CAD build for the part. Positions are in the model's coordinates, mm. Face numbers are marked on the shaded views. A direction names the side the tool comes from. Give positions to 0.01 mm unless a question says otherwise; leave off trailing zeros. Order: outer loops, then holes, each group sorted by start corner. A loop starts at its lowest first (then second) coordinate and runs counter-clockwise, first axis right, second up. Notation, with made-up numbers: (21, -1.75) -> (46, -1.75) arc R19 cw to (46, 21.25) -> close; hole circle Ø6 at (-7.75, 21). An arc over 180 degrees is marked (long way). Use one line per item in the form item = value. Start each with the question number.
1) Drop flat-ended pins along their axis: P1, Ø3, axis at x = 2, y = 8, coming from the -Z side (3 decimals); P2, Ø5, axis at x = 3.5, z = 61, coming from the +Y side; P3, Ø10, axis at y = -8, z = 22.5, coming from the +X side. Give the stop position or say it passes through.
2) Cut at D-D, the plane x = -9.25. Give the cut face in (y, z) (3 decimals).
3) Tool access for the marked faces 1, 2 and 3: list every direction of +Z, -Z, +X, -X, +Y, -Y with a clear straight run to the whole face (end or side of a thin tool).
4) Cut at C-C, the plane z = 24.5. Give the cut face in (x, y) (1 decimal), and give its area (3 significant figures).
5) Cut at B-B, the plane y = 0. Give the cut face in (x, z) (1 decimal).
6) Probe line 1 (Z direction, x = -2, y = 4.5) (3 decimals); line 2 (Z direction, x = -6.5, y = 0.5) (3 decimals); line 3 (Y direction, x = 0.5, z = 11.5). List the from-to ranges inside material, lowest first.
7) Cut at A-A, the plane x = 0. Give the cut face in (y, z) (1 decimal), and give its area (3 significant figures).
from build123d import *

# Parameters (mm, degrees)
F0_R     = 11.1125
F1_DEPTH = 76.2
F2_R     = 15.748
F3_DEPTH = 9.525
F4_R     = 6
F5_DEPTH = 25.4
F6_R     = 6
F6_R_2   = 4.8895
F7_DEPTH = 2.794
F8_W     = 13.440132
F8_H     = 49.0506
F9_DEPTH = 85.726


with BuildPart() as f1:
    # F0 (on Top) → F1 (new body)
    with BuildSketch(Plane.XY):
        Circle(F0_R)
    extrude(amount=F1_DEPTH)

    # F2 (on face) → F3 (join)
    with BuildSketch(Plane(origin=(0, 0, 0), x_dir=(1, 0, 0), z_dir=(0, 0, -1))):
        Circle(F2_R)
    extrude(amount=F3_DEPTH)

    # F4 (on face) → F5 (join)
    with BuildSketch(Plane(origin=(0, 0, -9.525), x_dir=(1, 0, 0), z_dir=(0, 0, -1))):
        Circle(F4_R)
    extrude(amount=F5_DEPTH)

    # F6 (on face) → F7 (cut)
    with BuildSketch(Plane(origin=(0, 0, -9.525), x_dir=(1, 0, 0), z_dir=(0, 0, -1))):
        Circle(F6_R)
        Circle(F6_R_2, mode=Mode.SUBTRACT)
    extrude(amount=F7_DEPTH, mode=Mode.SUBTRACT)

    # F8 (on face) → F9 (cut, through all)
    with BuildSketch(Plane(origin=(0, 0, -9.525), x_dir=(1, 0, 0), z_dir=(0, 0, -1))):
        with Locations((-19.420066, 0)):
            Rectangle(F8_W, F8_H)
        with Locations((19.420066, 0)):
            Rectangle(F8_W, F8_H)
    extrude(amount=-F9_DEPTH, mode=Mode.SUBTRACT)


solid = f1.part
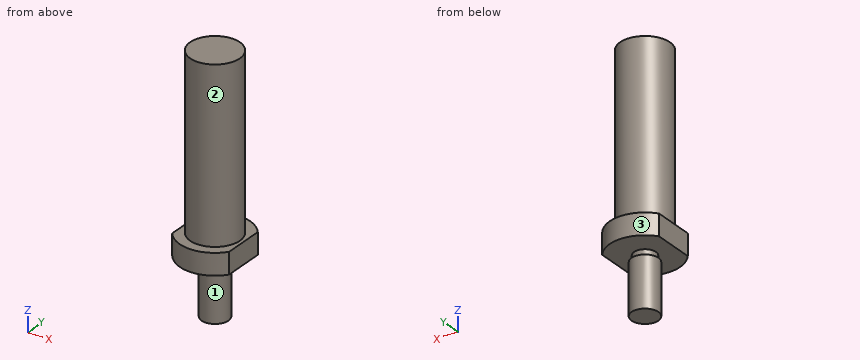
Result:
q1.P1 = -9.525
q1.P2 = 11.07
q1.P3 = 10.7
q2.outline = (-12.745, -9.525) -> (12.745, -9.525) -> (12.745, 0) -> (6.158, 0) -> (6.158, 76.2) -> (-6.158, 76.2) -> (-6.158, 0) -> (-12.745, 0) -> close
q3.face_1 = -Z
q3.face_2 = +Z
q3.face_3 = +Z, -Z, +Y
q4.outline = circle Ø22.2 at (0, 0)
q4.area = 388 mm²
q5.outline = (-12.7, -9.5) -> (-4.9, -9.5) -> (-4.9, -12.3) -> (-6, -12.3) -> (-6, -34.9) -> (6, -34.9) -> (6, -12.3) -> (4.9, -12.3) -> (4.9, -9.5) -> (12.7, -9.5) -> (12.7, 0) -> (11.1, 0) -> (11.1, 76.2) -> (-11.1, 76.2) -> (-11.1, 0) -> (-12.7, 0) -> close
q6.line_1 = -34.925 to -12.319, -9.525 to 76.2
q6.line_2 = -9.525 to 76.2
q6.line_3 = -11.1 to 11.1
q7.outline = (-15.7, -9.5) -> (-4.9, -9.5) -> (-4.9, -12.3) -> (-6, -12.3) -> (-6, -34.9) -> (6, -34.9) -> (6, -12.3) -> (4.9, -12.3) -> (4.9, -9.5) -> (15.7, -9.5) -> (15.7, 0) -> (11.1, 0) -> (11.1, 76.2) -> (-11.1, 76.2) -> (-11.1, 0) -> (-15.7, 0) -> close
q7.area = 2,290 mm²
